Verification items for this drawing (mm, ordinates from the low corner). Give positions to 0.01 mm unless a question says otherwise; leave off trailing zeros. Write each loop counter-clockwise with the first axis right and the second up, starting at its lowest first coordinate (ties: lowest second). Pieces come first, ordered by that corner, then holes. Notation, with made-up numbers: M 55.5,64.25 L 101.5,64.25 A30 ccw 101.5,86.25 Z; hole C 57,-29.5 d7. An arc over 180 degrees is marked long. Write each question's results on one line, items separated by ' | '.
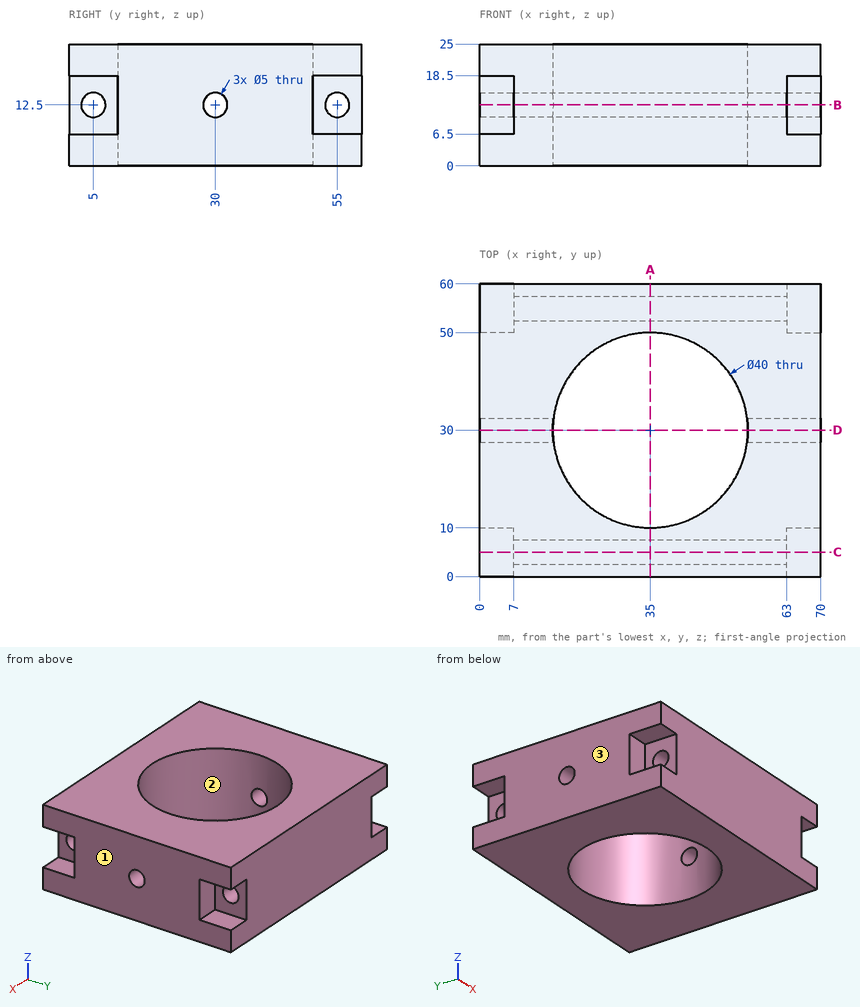
Q1. Section check C-C (y = 5). Enter the section's corners in (x, z), then the cut area to 3 significant figures.
Answer key:
outline: M 0,0 L 70,0 L 70,6.5 L 63,6.5 L 63,10 L 7,10 L 7,6.5 L 0,6.5 Z; M 0,18.5 L 7,18.5 L 7,15 L 63,15 L 63,18.5 L 70,18.5 L 70,25 L 0,25 Z | area: 1,300 mm2
Q2. Material ranges on probe 1 along Y at (x, z) = (61.75, 12.5); probe 2 along Z at (x, y) = (66.5, 30); probe 3 along X at (y, z) = (30, 5.5), recorded low to high. Write a range as [from, to].
Answer key:
probe 1: y = [0, 2.5], [7.5, 27.5], [32.5, 52.5], [57.5, 60] | probe 2: z = [0, 10], [15, 25] | probe 3: x = [0, 15], [55, 70]
Q3. Section check B-B (z = 12.5). Enter the section's corners in (x, y).
Answer key:
outline: M 0,10 L 7,10 L 7,7.5 L 63,7.5 L 63,10 L 70,10 L 70,27.5 L 54.84,27.5 A20 cw 15.16,27.5 L 0,27.5 Z; M 0,32.5 L 15.16,32.5 A20 cw 54.84,32.5 L 70,32.5 L 70,50 L 63,50 L 63,52.5 L 7,52.5 L 7,50 L 0,50 Z; M 7,0 L 63,0 L 63,2.5 L 7,2.5 Z; M 7,57.5 L 63,57.5 L 63,60 L 7,60 Z
Q4. Section check A-A (x = 35). Enter the section's corners in (y, z), then the cut area to 3 significant figures.
Answer key:
outline: M 0,0 L 10,0 L 10,25 L 0,25 Z; M 50,0 L 60,0 L 60,25 L 50,25 Z; hole C 5,12.5 d5; hole C 55,12.5 d5 | area: 461 mm2
Q5. Section check D-D (y = 30). Enter the section's corners in (x, z).
Answer key:
outline: M 0,0 L 15,0 L 15,10 L 0,10 Z; M 0,15 L 15,15 L 15,25 L 0,25 Z; M 55,0 L 70,0 L 70,10 L 55,10 Z; M 55,15 L 70,15 L 70,25 L 55,25 Z
Q6. Release check for a two-part mould opening along X. For the marked faces 1, 2 and 3 record: released by +X, released by -X, zero draft, split by the parting line, or undercut.
Answer key:
face 1: released by +X | face 2: undercut | face 3: released by -X
Q7. Depth check by flat-ended pin: P1, Ø5.5, axis at x = 67, z = 10.5, coming from the +Y side; P2, Ø6, axis at y = 5, z = 12.5, coming from the -X side. Enter the tip coordinate at first touch or a pass-through.
Answer key:
P1: stops at y = 50 | P2: stops at x = 7
